```python
from build123d import *

# Parameters (mm, degrees)
EXTRUDE_1_DEPTH     = 3
SKETCH_2_W          = 42
SKETCH_2_H          = 10.974531836
CUT_EXTRUDE_1_DEPTH = 3
SKETCH_3_W          = 15.635920588
SKETCH_3_H          = 9
SKETCH_3_R          = 1.5
EXTRUDE_2_DEPTH     = 3
EXTRUDE_7_DEPTH     = 1
SKETCH_5_W          = 42
SKETCH_5_H          = 8
CUT_EXTRUDE_2_DEPTH = 1
SKETCH_6_R          = 1.5
CUT_EXTRUDE_3_DEPTH = 1


with BuildPart() as part:
    # 草图1 → 凸台-拉伸1 (new body)
    with BuildSketch(Plane.XY):
        with BuildLine():
            Line((36.635920588, -39.974531836), (-36.635920588, -39.974531836))
            add(Edge.make_bspline(
                [(-36.635920588, -39.974531836), (-34.121545097, -16.704406605), (-43.139592985, 2.527664637), (-62.878950173, 15.795774826)],
                knots=[0, 0, 0, 0, 0.89990839, 0.89990839, 0.89990839, 0.89990839], degree=3))
            ThreePointArc((-62.878950173, 15.795774826), (-63.630739893, 18.171500647), (-61.483579663, 19.436002094))
            ThreePointArc((-61.483579663, 19.436002094), (-36.207222823, 9.690254792), (-17.793837687, -10.179849722))
            ThreePointArc((-17.793837687, -10.179849722), (0, -20.5), (17.793837687, -10.179849722))
            ThreePointArc((17.793837687, -10.179849722), (36.207222823, 9.690254792), (61.483579663, 19.436002094))
            ThreePointArc((61.483579663, 19.436002094), (63.630739893, 18.171500647), (62.878950173, 15.795774826))
            add(Edge.make_bspline(
                [(36.635920588, -39.974531836), (34.121545097, -16.704406605), (43.139592985, 2.527664637), (62.878950173, 15.795774826)],
                knots=[0, 0, 0, 0, 0.89990839, 0.89990839, 0.89990839, 0.89990839], degree=3))
        make_face()
    extrude(amount=EXTRUDE_1_DEPTH)

    # 草图2 → 切除-拉伸1 (cut)
    with BuildSketch(Plane(origin=(0, 0, 0), x_dir=(-1, 0, 0), z_dir=(0, 0, -1))):
        with Locations((0, -34.487265918)):
            Rectangle(SKETCH_2_W, SKETCH_2_H)
    extrude(amount=-CUT_EXTRUDE_1_DEPTH, mode=Mode.SUBTRACT)

    # 草图3 → 凸台-拉伸2 (add)
    # profile 1 of 2: a face of its own
    with BuildSketch(Plane(origin=(0, 0, 0), x_dir=(-1, 0, 0), z_dir=(0, 0, -1))):
        with Locations((-28.817960294, -44.474531836)):
            Rectangle(SKETCH_3_W, SKETCH_3_H)
        with Locations((-31, -44)):
            Circle(SKETCH_3_R, mode=Mode.SUBTRACT)
    # profile 2 of 2: a face of its own
    with BuildSketch(Plane(origin=(0, 0, 0), x_dir=(-1, 0, 0), z_dir=(0, 0, -1))):
        with Locations((28.817960294, -44.474531836)):
            Rectangle(SKETCH_3_W, SKETCH_3_H)
        with Locations(Location((31, -44, 0), (0, 0, 180))):
            Circle(SKETCH_3_R, mode=Mode.SUBTRACT)
    extrude(amount=-EXTRUDE_2_DEPTH)

    # 草图4 → 凸台-拉伸7 (add)
    with BuildSketch(Plane.XY.offset(3)):
        with BuildLine():
            Line((-21, -29), (-21, -21))
            Line((-21, -21), (21, -21))
            Line((21, -21), (21, -29))
            Line((21, -29), (21, -48.974531836))
            Line((21, -48.974531836), (36.635920588, -48.974531836))
            Line((36.635920588, -48.974531836), (36.635920588, -39.974531836))
            add(Edge.make_bspline(
                [(36.635920588, -39.974531836), (34.121545097, -16.704406605), (43.139592985, 2.527664637), (62.878950173, 15.795774826)],
                knots=[0, 0, 0, 0, 0.89990839, 0.89990839, 0.89990839, 0.89990839], degree=3))
            ThreePointArc((62.878950173, 15.795774826), (63.630739893, 18.171500647), (61.483579663, 19.436002094))
            ThreePointArc((61.483579663, 19.436002094), (36.207222823, 9.690254792), (17.793837687, -10.179849722))
            ThreePointArc((17.793837687, -10.179849722), (0, -20.5), (-17.793837687, -10.179849722))
            ThreePointArc((-17.793837687, -10.179849722), (-36.207222823, 9.690254792), (-61.483579663, 19.436002094))
            ThreePointArc((-61.483579663, 19.436002094), (-63.630739893, 18.171500647), (-62.878950173, 15.795774826))
            add(Edge.make_bspline(
                [(-62.878950173, 15.795774826), (-43.139592985, 2.527664637), (-34.121545097, -16.704406605), (-36.635920588, -39.974531836)],
                knots=[0, 0, 0, 0, 0.89990839, 0.89990839, 0.89990839, 0.89990839], degree=3))
            Line((-36.635920588, -39.974531836), (-36.635920588, -48.974531836))
            Line((-36.635920588, -48.974531836), (-21, -48.974531836))
            Line((-21, -48.974531836), (-21, -29))
        make_face()
    extrude(amount=EXTRUDE_7_DEPTH)

    # 草图5 → 切除-拉伸2 (cut)
    with BuildSketch(Plane.XY.offset(3)):
        with Locations((0, -25)):
            Rectangle(SKETCH_5_W, SKETCH_5_H)
    extrude(amount=-CUT_EXTRUDE_2_DEPTH, mode=Mode.SUBTRACT)

    # 草图6 → 切除-拉伸3 (cut)
    with BuildSketch(Plane(origin=(0, 0, 3), x_dir=(-1, 0, 0), z_dir=(0, 0, -1))):
        with Locations((-31, -44)):
            Circle(SKETCH_6_R)
        with Locations((31, -44)):
            Circle(SKETCH_6_R)
    extrude(amount=-CUT_EXTRUDE_3_DEPTH, mode=Mode.SUBTRACT)


solid = part.part
```
Geometry: final body of the model. Coordinates: model frame, mm. A direction names the side the tool comes from. Give positions to 0.01 mm unless a question says otherwise; leave off trailing zeros. Order: outer loops, then holes, each group sorted by start corner. A loop starts at its lowest first (then second) coordinate and runs counter-clockwise, first axis right, second up. Notation, with made-up numbers: (32, -39) -> (91, -39) arc R21 ccw to (91, -2) -> close; hole circle Ø5 at (24, -29.5). An arc over 180 degrees is marked (long way). Write each question's results on one line, items separated by ' | '. Start each with the question number.
1) First-contact query: pin 1 (2.5 mm diameter, centred on x = 31, y = -44, fed in from +Z); pin 2 (1.6 mm diameter, centred on x = -5, z = 3, fed in from -Y); pin 3 (2 mm diameter, centred on x = 1.5, z = 1, fed in from -Y); pin 4 (1.2 mm diameter, centred on y = -45.5, z = 1.5, fed in from +X). Flat tips, straight axial feed; report the tip coordinate or a pass-through.
2) Section C-C (x = -11.5). Return loops of the section in (y, z).
3) Section A-A (z = 1). Count the separate pieces of the cut face and the enclosed holes in it, then the cut area to 3 significant figures.
4) Line query: line 1 (X direction, y = -45, z = 0.4); line 2 (Z direction, x = -8, y = -27); line 3 (X direction, y = -19, z = 2.6). Output: solid intervals per line, ascending. Write a range as from..to.
5) Set-up query: faces 1 (the flat face through (-21, -38, 2)), 2 (the cylindrical face through (36.52, 9.9, 1.97)), 3 (the flat face through (-36.636, -44, 2)). Return all of +Z, -Z, +X, -X, +Y, -Y with unobstructed straight access to the full face (end or side cutting, diameter ignored); none if empty.
6) Section B-B (x = 31). Return loops of the section in (y, z), then the cut area to 3 significant figures.
Calculated:
1) pin 1: through | pin 2: y = -21 | pin 3: y = -29 | pin 4: x = 36.64
2) outline: (-29, 0) -> (-16.97, 0) -> (-16.97, 4) -> (-21, 4) -> (-21, 2) -> (-29, 2) -> close
3) separate pieces: 1 | enclosed holes: 2 | area: 2,890 mm2
4) line 1: -36.64..-32.12, -29.88..-21, 21..29.88, 32.12..36.64 | line 2: 0..2 | line 3: -37.72..-7.7, 7.7..37.72
5) face 1: +Z, -Y | face 2: +Z, -Z, +Y | face 3: +Z, -Z, -X, -Y
6) outline: (-48.97, 0) -> (-45.5, 0) -> (-45.5, 4) -> (-48.97, 4) -> close; (-42.5, 0) -> (5.73, 0) -> (5.73, 4) -> (-42.5, 4) -> close | area: 207 mm2
